Geometry check sheet. Reference: the model listing, model coordinates, mm. Face numbers are marked on the shaded views. A direction names the side the tool comes from. Round coordinates to 2 decimals unless told otherwise and drop trailing zeros. Loops run counter-clockwise (first coordinate to the right, second up) from the corner with the lowest first, then second, coordinate; pieces in that order, holes last.
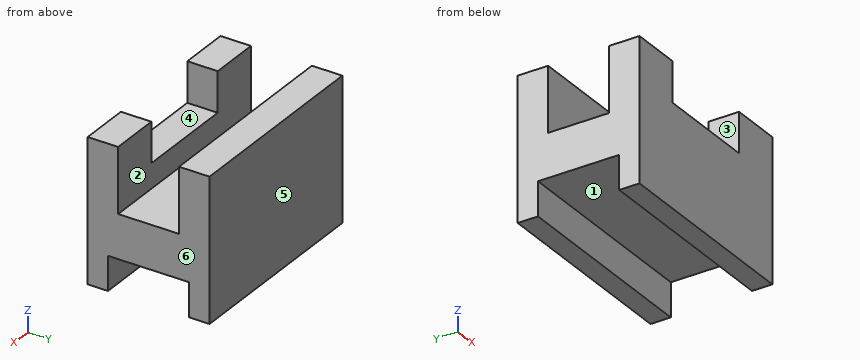
```python
from build123d import *

# Parameters (mm, degrees)
F0_W     = 63.5
F0_H     = 44.45
F1_DEPTH = 38.1
F3_W     = 19.05
F3_H     = 20.2448921431
F4_DEPTH = 63.5
F2_W     = 31.75
F2_H     = 12.5393269187
F5_DEPTH = 25.4
F6_W     = 25.4
F6_H     = 10.5997411049
F7_DEPTH = 63.5


with BuildPart() as f1:
    # F0 (on Front) → F1 (new body)
    with BuildSketch(Plane.XZ):
        Rectangle(F0_W, F0_H)
    extrude(amount=F1_DEPTH)

    # F3 (on face) → F4 (cut)
    with BuildSketch(Plane.YZ.offset(31.75)):
        with Locations((-19.05, 12.1025539285)):
            Rectangle(F3_W, F3_H)
    extrude(amount=-F4_DEPTH, mode=Mode.SUBTRACT)

    # F2 (on face) → F5 (cut)
    with BuildSketch(Plane.XZ.offset(38.1)):
        with Locations((0, 15.9553365407)):
            Rectangle(F2_W, F2_H)
    extrude(amount=-F5_DEPTH, mode=Mode.SUBTRACT)

    # F6 (on face) → F7 (cut)
    with BuildSketch(Plane.YZ.offset(31.75)):
        with Locations((-19.05, -16.9251294475)):
            Rectangle(F6_W, F6_H)
    extrude(amount=-F7_DEPTH, mode=Mode.SUBTRACT)


solid = f1.part
```
1) Sectioned sample at B-B, the plane z = -18. Record the cut outline in (x, y).
Report:
outline: (-31.75, -38.1) - (31.75, -38.1) - (31.75, -31.75) - (-31.75, -31.75) - close; (-31.75, -6.35) - (31.75, -6.35) - (31.75, 0) - (-31.75, 0) - close
2) Scan lines: line 1 along Y through (x, z) = (2, 8) (3 decimals); line 2 along X through (y, z) = (-33, 17) (3 decimals); line 3 along Z through (x, y) = (23, -8) (3 decimals). Record each from-to range of solid material in increasing order.
Report:
line 1: y = -38.1 to -28.575, -9.525 to 0
line 2: x = -31.75 to -15.875, 15.875 to 31.75
line 3: z = -11.625 to 22.225
3) Mould release check, pull along X, two halves, no side actions. Record for the marked faces 4, 5 and 6: +X half, -X half, draft (parallel to the pull), parting line (faces both ways), or undercut.
Report:
face 4: undercut
face 5: draft
face 6: +X half
4) Sectioned sample at C-C, the plane x = 24. Record the cut outline in (y, z) (3 decimals), then the cut area to 3 significant figures.
Report:
outline: (-38.1, -22.225) - (-31.75, -22.225) - (-31.75, -11.625) - (-6.35, -11.625) - (-6.35, -22.225) - (0, -22.225) - (0, 22.225) - (-9.525, 22.225) - (-9.525, 1.98) - (-28.575, 1.98) - (-28.575, 22.225) - (-38.1, 22.225) - close
area: 1,040 mm2
5) Sectioned sample at A-A, the plane z = 10.5. Record the cut outline in (x, y) (3 decimals).
Report:
outline: (-31.75, -38.1) - (-15.875, -38.1) - (-15.875, -28.575) - (-31.75, -28.575) - close; (-31.75, -9.525) - (31.75, -9.525) - (31.75, 0) - (-31.75, 0) - close; (15.875, -38.1) - (31.75, -38.1) - (31.75, -28.575) - (15.875, -28.575) - close
6) Sectioned sample at D-D, the plane y = -7.5. Record the cut outline in (x, z) (3 decimals), then the cut area to 3 significant figures.
Report:
outline: (-31.75, -11.625) - (31.75, -11.625) - (31.75, 22.225) - (-31.75, 22.225) - close
area: 2,150 mm2
7) Gauge pin test, flat ends, axial feed: pin 1 (8 mm diameter, centred on x = 12, y = -23.5, fed in from -Z); pin 2 (5 mm diameter, centred on x = -7.5, z = 13, fed in from -Y) (3 decimals); pin 3 (3 mm diameter, centred on x = 3, y = -32, fed in from +Z). Record the tip position at first contact, or that the pin passes through.
Report:
pin 1: stops at z = -11.63
pin 2: stops at y = -9.525
pin 3: stops at z = 9.69
8) Access from +Z, -Z, +X, -X, +Y, -Y to the whole of each face (thin tool, end or side, straight path). Record for the marked faces 1, 2 and 3.
Report:
face 1: -Z, +X, -X
face 2: +Z, +X, -X
face 3: +Z, -Y
